Read the model definition and answer for the solid it produces. Units are mm, in the model's axes. Round coordinates to 2 decimals unless told otherwise and drop trailing zeros. Order: outer loops, then holes, each group sorted by start corner. A loop starts at its lowest first (then second) coordinate and runs counter-clockwise, first axis right, second up. Notation, with made-up numbers: (-27.75, 63) -> (-6.75, 63) arc R17 cw to (-6.75, 74) -> close; hole circle Ø4 at (85, 24.5). An arc over 180 degrees is marked (long way). One line per item, written item: value. Start each with the question number.
1. Section C-C (x = 26.5) is taken. Give the vertices of the cut face in (y, z), then the cut area to 3 significant figures.
2. Section B-B (x = 0) is taken. Give the vertices of the cut face in (y, z), then the cut area to 3 significant figures.
3. Section A-A (y = 0) is taken. Give the vertices of the cut face in (x, z), then the cut area to 4 significant figures.
4. Consider line 1 (Y direction, x = 0, z = 2.25); line 2 (X direction, y = 6.5, z = 0.9); line 3 (X direction, y = 7.5, z = 0.8). Determine where each line is inside the solid, lowest interval first.
5. Flat-ended cylindrical pins translate along their axes: pin 1 Ø1.5 at (x, z) = (40.5, 1.5) entering from -Y; pin 2 Ø1 at (y, z) = (-6.5, 4) entering from -X; pin 3 Ø2.5 at (x, z) = (-27, 2) entering from +Y. Find the tip coordinate at first contact, or state that the pin passes through.
from build123d import *

# Parameters (mm, degrees)
F0_R     = 3.25
F1_DEPTH = 5
F2_R     = 5


with BuildPart() as f1:
    # F0 (on Top) → F1 (new body)
    with BuildSketch(Plane.XY):
        Polygon((-80, 10), (-80, -10), (-60, -10), (-55, -5), (-15.177652, -5), (-10, -10), (10, -10), (15.177652, -5), (55, -5), (60, -10), (80, -10), (80, 10), (60, 10), (55, 5), (15.177652, 5), (10, 10), (-10, 10), (-15.177652, 5), (-55, 5), (-60, 10), align=None)
        Circle(F0_R, mode=Mode.SUBTRACT)
    extrude(amount=F1_DEPTH)

    # F2
    f2_edges = [f1.edges().sort_by_distance(p)[0] for p in [
        (-80, -10, 2.5),
        (-55, -5, 2.5),
        (-10, -10, 2.5),
        (10, -10, 2.5),
        (15.177652, -5, 2.5),
        (60, -10, 2.5),
        (80, -10, 2.5),
        (80, 10, 2.5),
        (60, 10, 2.5),
        (10, 10, 2.5),
        (15.177652, 5, 2.5),
        (-55, 5, 2.5),
        (-60, 10, 2.5),
        (-80, 10, 2.5),
        (-10, 10, 2.5),
        (55, 5, 2.5),
        (-15.177652, 5, 2.5),
        (-15.177652, -5, 2.5),
        (55, -5, 2.5),
        (-60, -10, 2.5),
    ]]
    fillet(f2_edges, radius=F2_R)


solid = f1.part
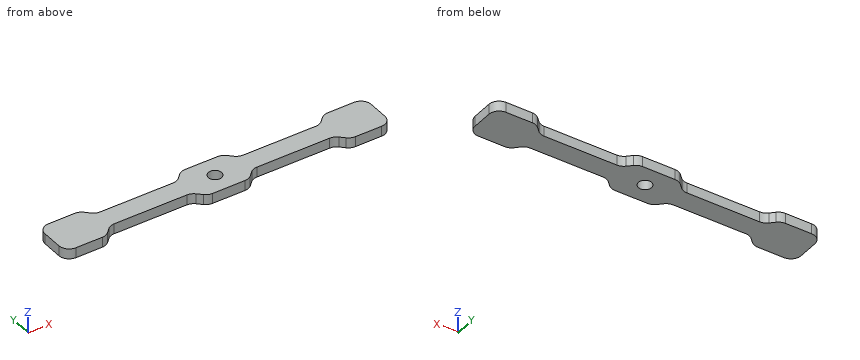
Answer:
1. outline: (-5, 0) -> (5, 0) -> (5, 5) -> (-5, 5) -> close
1. area: 50.0 mm^2
2. outline: (-10, 0) -> (-3.25, 0) -> (-3.25, 5) -> (-10, 5) -> close; (3.25, 0) -> (10, 0) -> (10, 5) -> (3.25, 5) -> close
2. area: 67.5 mm^2
3. outline: (-80, 0) -> (-3.25, 0) -> (-3.25, 5) -> (-80, 5) -> close; (3.25, 0) -> (80, 0) -> (80, 5) -> (3.25, 5) -> close
3. area: 767.5 mm^2
4. line 1: -10 to -3.25, 3.25 to 10
4. line 2: -79.77 to -56.5, -13.62 to 13.62, 56.5 to 79.77
4. line 3: -79.33 to -57.5, -12.59 to 12.59, 57.5 to 79.33
5. pin 1: y = -5
5. pin 2: x = -79.9
5. pin 3: y = 5
